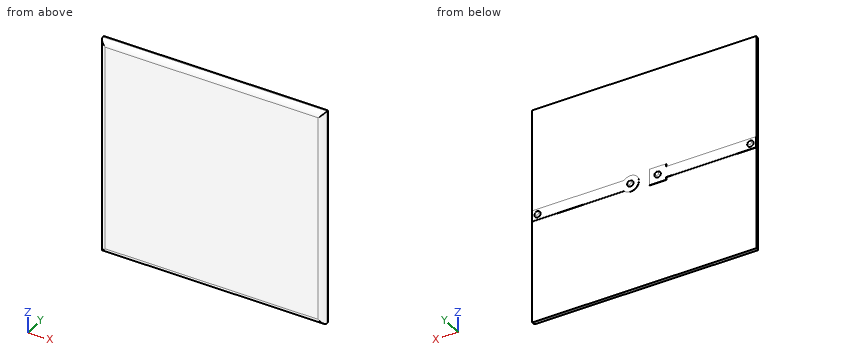
```python
from build123d import *

# Parameters (mm, degrees)
SKETCH_1_W      = 79.7
SKETCH_1_H      = 79.7
EXTRUDE_1_DEPTH = 2.5
FILLET_1_R      = 2
SKETCH_2_W      = 37
SKETCH_2_H      = 4
EXTRUDE_2_DEPTH = 0.1
SKETCH_3_R      = 3
SKETCH_3_W      = 6
SKETCH_3_H      = 6
EXTRUDE_3_DEPTH = 0.1
SKETCH_4_R      = 1.1
EXTRUDE_4_DEPTH = 0.5
FILLET_2_R      = 0.5


with BuildPart() as part:
    # Эскиз1 → Бобышка-Вытянуть1 (new body)
    with BuildSketch(Plane(origin=(0, 0, 0), x_dir=(1, 0, 0), z_dir=(0, 1, 0))):
        Rectangle(SKETCH_1_W, SKETCH_1_H)
    extrude(amount=-EXTRUDE_1_DEPTH)

    # Скругление1
    fillet_1_edges = [part.edges().sort_by_distance(p)[0] for p in [
        (39.85, -2.5, 0),
        (0, -2.5, -39.85),
        (-39.85, -2.5, 0),
        (0, -2.5, 39.85),
    ]]
    fillet(fillet_1_edges, radius=FILLET_1_R)

    # Эскиз2 → Бобышка-Вытянуть2 (add)
    with BuildSketch(Plane(origin=(0, 0, 0), x_dir=(1, 0, 0), z_dir=(0, 1, 0))):
        with Locations((21.35, 0)):
            Rectangle(SKETCH_2_W, SKETCH_2_H)
        with Locations((-21.35, 0)):
            Rectangle(SKETCH_2_W, SKETCH_2_H)
    extrude(amount=EXTRUDE_2_DEPTH)

    # Эскиз3 → Бобышка-Вытянуть3 (add)
    with BuildSketch(Plane(origin=(0, 0, 0), x_dir=(1, 0, 0), z_dir=(0, 1, 0))):
        with Locations((4.85, 0)):
            Circle(SKETCH_3_R)
        with Locations((-4.85, 0)):
            Rectangle(SKETCH_3_W, SKETCH_3_H)
    extrude(amount=EXTRUDE_3_DEPTH)

    # Эскиз4 → Бобышка-Вытянуть4 (add)
    with BuildSketch(Plane(origin=(0, 0.1, 0), x_dir=(1, 0, 0), z_dir=(0, 1, 0))):
        with Locations(Location((4.85, 0, 0), (0, 0, 270))):
            Circle(SKETCH_4_R)
        with Locations(Location((-4.85, 0, 0), (0, 0, 270))):
            Circle(SKETCH_4_R)
        with Locations(Location((37.85, 0, 0), (0, 0, 270))):
            Circle(SKETCH_4_R)
        with Locations(Location((-37.85, 0, 0), (0, 0, 270))):
            Circle(SKETCH_4_R)
    extrude(amount=EXTRUDE_4_DEPTH)

    # Скругление2
    fillet_2_edges = [part.edges().sort_by_distance(p)[0] for p in [
        (4.85, 0.6, -1.1),
        (-4.85, 0.6, -1.1),
        (37.85, 0.6, -1.1),
        (-37.85, 0.6, -1.1),
    ]]
    fillet(fillet_2_edges, radius=FILLET_2_R - 0.0001)  # a hair under: the kernel refuses the full size


solid = part.part
```
Input: part model. Units: mm. Frame: model coordinates. Give positions to 0.01 mm unless a question says otherwise; leave off trailing zeros. Write each loop counter-clockwise with the first axis right and the second up, starting at its lowest first coordinate (ties: lowest second). Pieces come first, ordered by that corner, then holes. Notation, with made-up numbers: (60.5, 6) - (108.5, 6) arc R18 ccw to (108.5, 34) - close; hole circle Ø3 at (-32, 31.25). An arc over 180 degrees is marked (long way). Write item = value, one per line. Start each with the question number.
1. Section query B-B, the plane z = -30. Output: boundary loops of the cut face in (x, y).
2. Ray query, L1, parallel to Y at x = 10, z = -19; L2, parallel to Y at x = -30, z = 1; L3, parallel to X at y = -0.65, z = 9. Return the intervals inside material, ascending.
3. Section query A-A, the plane x = -25.5. Output: boundary loops of the cut face in (y, z).
4. First-contact query: pin 1 Ø3 at (x, z) = (-14.5, 0.5) entering from +Y. Flat tip, straight axial feed; report the tip coordinate or a pass-through.
5. Section query C-C, the plane y = -1.7. Output: boundary loops of the cut face in (x, z), then the cut area to 3 significant figures.
Check sheet entries:
q1.outline = (-39.85, -0.5) arc R2 ccw to (-37.85, -2.5) - (37.85, -2.5) arc R2 ccw to (39.85, -0.5) - (39.85, 0) - (-39.85, 0) - close
q2.L1 = -2.5 to 0
q2.L2 = -2.5 to 0.1
q2.L3 = -39.84 to 39.84
q3.outline = (-2.5, -37.85) arc R2 ccw to (-0.5, -39.85) - (0, -39.85) - (0, -2) - (0.1, -2) - (0.1, 2) - (0, 2) - (0, 39.85) - (-0.5, 39.85) arc R2 ccw to (-2.5, 37.85) - close
q4.pin_1 = 0.1
q5.outline = (-39.45, -39.45) - (39.45, -39.45) - (39.45, 39.45) - (-39.45, 39.45) - close
q5.area = 6,230 mm2
